```python
from build123d import *

# Parameters (mm, degrees)
SKETCH_W       = 31.75
SKETCH_H       = 31.75
SKETCH_W_2     = 26.2128
SKETCH_H_2     = 26.2128
PAD_DEPTH      = 152.4
PAD_DEPTH_BACK = 152.4
POCKET_DEPTH   = 31.75


with BuildPart() as part:
    # Sketch → Pad (new body, two sides)
    with BuildSketch(Plane.YZ) as pad_sk:
        Rectangle(SKETCH_W, SKETCH_H)
        Rectangle(SKETCH_W_2, SKETCH_H_2, mode=Mode.SUBTRACT)
    extrude(amount=PAD_DEPTH)
    extrude(pad_sk.sketch, amount=-PAD_DEPTH_BACK)

    # Sketch001 → Pocket (cut)
    with BuildSketch(Plane(origin=(0, -15.875, 0), x_dir=(0, 0, -1), z_dir=(0, -1, 0))):
        Polygon((-15.875, 152.4), (15.875, 152.4), (15.875, 126.371257), align=None)
    pocket = extrude(amount=-POCKET_DEPTH, mode=Mode.SUBTRACT)

    # Mirrored: Pocket across Sketch001 H_Axis
    add(pocket.mirror(Plane(origin=(0, -15.875, 0), x_dir=(0, -1, 0), z_dir=(1, 0, 0))), mode=Mode.SUBTRACT)


solid = part.part
```
Verification items for the finished model (mm, model axes). A direction names the side the tool comes from. Coordinates: 2 decimals unless noted, no trailing zeros. Order: outer loops, then holes, each group sorted by start corner. A loop starts at its lowest first (then second) coordinate and runs counter-clockwise, first axis right, second up. Notation, with made-up numbers: (58, -38.75) - (107, -38.75) arc R21 ccw to (107, -2.75) - close; hole circle Ø8 at (14.5, 55). An arc over 180 degrees is marked (long way). Return JSON: item names as keys, results as strings.
(1) Go/stop test with a flat-tipped pin: pin 1 (8 mm diameter, centred on y = -4, z = 12, fed in from -X). Record where the tip stops, or that it passes through.
Filled sheet:
{"pin 1": "stops at x = -152.4"}
(2) Section check C-C, the plane z = -6. Record the cut outline in (x, y) (3 decimals).
Filled sheet:
{"outline": "(-134.467, -15.875) - (134.467, -15.875) - (134.467, -13.106) - (-134.467, -13.106) - close; (-134.467, 13.106) - (134.467, 13.106) - (134.467, 15.875) - (-134.467, 15.875) - close"}
(3) Section check A-A, the plane x = 119. Record the cut outline in (y, z) (3 decimals), and give its area (3 significant figures).
Filled sheet:
{"outline": "(-15.875, -15.875) - (15.875, -15.875) - (15.875, 15.875) - (-15.875, 15.875) - close; hole (-13.106, -13.106) - (13.106, -13.106) - (13.106, 13.106) - (-13.106, 13.106) - close", "area": "321 mm^2"}
(4) Section check D-D, the plane x = -133. Record the cut outline in (y, z) (3 decimals).
Filled sheet:
{"outline": "(-15.875, -7.789) - (-13.106, -7.789) - (-13.106, 13.106) - (13.106, 13.106) - (13.106, -7.789) - (15.875, -7.789) - (15.875, 15.875) - (-15.875, 15.875) - close"}
(5) Thickness scan on line 1 along Z through (x, y) = (84, -10) (3 decimals); line 2 along Z through (x, y) = (135, 14) (3 decimals). Record the ranges inside material, lowest first.
Filled sheet:
{"line 1": "z = -15.875 to -13.106, 13.106 to 15.875", "line 2": "z = -5.35 to 15.875"}
(6) Access from +Z, -Z, +X, -X, +Y, -Y to the whole of each face (thin tool, end or side, straight path). Record for faces 4 (the flat face through (2, -15.875, 0)), 5 (the flat face through (2, 0, -13.106)).
Filled sheet:
{"face 4": "+Z, -Z, +X, -X, -Y", "face 5": "+X, -X"}
(7) Mould release check, pull along Y, two halves, no side actions. Record for faces 1 (the flat face through (2, 0, 13.106)), 2 (the flat face through (139.203, 13.889, -0.222)), 3 (the flat face through (2, 15.875, 0)): pulls with the +Y half, pulls with the -Y half, needs draft (parallel to the pull), parting line crosses it, or undercut.
Filled sheet:
{"face 1": "undercut", "face 2": "needs draft", "face 3": "pulls with the +Y half"}
(8) Section check B-B, the plane y = -6.5. Record the cut outline in (x, z) (3 decimals), and give its area (3 significant figures).
Filled sheet:
{"outline": "(-152.4, 15.875) - (-150.13, 13.106) - (150.13, 13.106) - (152.4, 15.875) - close; (-128.641, -13.106) - (-126.371, -15.875) - (126.371, -15.875) - (128.641, -13.106) - close", "area": "1,540 mm^2"}
